The listing builds one solid part. Answer for the finished solid, in the listing's coordinates (mm). A direction names the side the tool comes from. Give positions to 0.01 mm unless a question says otherwise; leave off trailing zeros. Write each loop counter-clockwise with the first axis right and the second up, starting at its lowest first coordinate (ties: lowest second). Pieces come first, ordered by that corner, then holes. Notation, with made-up numbers: M 42,-9.5 L 64,-9.5 A17 ccw 64,1.5 Z; hole C 47,-19 d3. An arc over 180 degrees is marked long. Answer as a JSON object with one key per item and string values.
```python
from build123d import *

# Parameters (mm, degrees)
SKETCH1_W                 = 30
SKETCH1_H                 = 28
SKETCH1_R                 = 11
BOSS_EXTRUDE1_DEPTH       = 7
SKETCH2_W                 = 5
SKETCH2_H                 = 2.5
BOSS_EXTRUDE2_DEPTH       = 13
CHAMFER2_SIZE             = 2
BOSS_EXTRUDE6_DEPTH       = 2.5
CHAMFER3_SIZE             = 2
CHAMFER4_SIZE             = 2
BOSS_EXTRUDE4_DEPTH       = 2.5
CHAMFER6_SIZE             = 2.5
CHAMFER7_SIZE             = 7
CHAMFER7_SIZE_2           = 13.165085257
SKETCH7_R                 = 1.5
CUT_EXTRUDE2_DEPTH        = 6.4
CUT_EXTRUDE3_START        = -3
SKETCH9_R                 = 1.5
CUT_EXTRUDE3_DEPTH        = 3
SKETCH10_W                = 5.5
SKETCH10_H                = 3
CUT_EXTRUDE4_DEPTH        = 5.6
CUT_EXTRUDE5_START        = -30
SKETCH10_2_W              = 5.5
SKETCH10_2_H              = 3
CUT_EXTRUDE5_DEPTH        = 5.6
F_1_0MM_DOWEL_HOLE1_D     = 3
F_1_0MM_DOWEL_HOLE1_DEPTH = 7.098709071
F_1_0MM_DOWEL_HOLE1_TIP   = 0.901290929
BOSS_EXTRUDE7_START       = 3.5
SKETCH17_R                = 1.5
BOSS_EXTRUDE7_DEPTH       = 3.5


with BuildPart() as part:
    # Sketch1 → Boss-Extrude1 (new body)
    with BuildSketch(Plane.XY):
        Rectangle(SKETCH1_W, SKETCH1_H)
        Circle(SKETCH1_R, mode=Mode.SUBTRACT)
    extrude(amount=BOSS_EXTRUDE1_DEPTH)

    # Sketch2 → Boss-Extrude2 (add)
    with BuildSketch(Plane(origin=(0, 0, 0), x_dir=(-1, 0, 0), z_dir=(0, 0, -1))):
        with Locations((-12.5, -12.75)):
            Rectangle(SKETCH2_W, SKETCH2_H)
        with Locations((12.5, -12.75)):
            Rectangle(SKETCH2_W, SKETCH2_H)
    extrude(amount=BOSS_EXTRUDE2_DEPTH)

    # Chamfer2
    chamfer2_edges = [part.edges().sort_by_distance(p)[0] for p in [
        (-10, -12.75, 0),
        (10, -12.75, 0),
    ]]
    chamfer(chamfer2_edges, length=CHAMFER2_SIZE)

    # Sketch5 → Boss-Extrude6 (add)
    with BuildSketch(Plane.XZ.offset(14)):
        Polygon((-10, -2), (-10, -7.5), (10, -7.5), (10, -2), (8, 0), (-8, 0), align=None)
    extrude(amount=-BOSS_EXTRUDE6_DEPTH)

    # Chamfer3
    chamfer3_edges = [part.edges().sort_by_distance(p)[0] for p in [
        (15, 0, 7),
    ]]
    chamfer(chamfer3_edges, length=CHAMFER3_SIZE)

    # Chamfer4
    chamfer4_edges = [part.edges().sort_by_distance(p)[0] for p in [
        (-15, 0, 7),
    ]]
    chamfer(chamfer4_edges, length=CHAMFER4_SIZE)

    # Sketch4 → Boss-Extrude4 (add)
    with BuildSketch(Plane(origin=(0, 0, 0), x_dir=(-1, 0, 0), z_dir=(0, 0, -1))):
        Polygon((-15, 0), (15, 11.5), (15, 14), (-15, 14), align=None)
    extrude(amount=BOSS_EXTRUDE4_DEPTH)

    # Chamfer6
    # the kernel refuses this chamfer: 2.5 mm, written as the material it adds along each edge
    with BuildSketch(Plane(origin=(21.003247512, -2.30124488, 0), x_dir=(-0.3578006820796162, -0.9333930836859554, 0.02749587661058638), z_dir=(-0.9337461173020497, 0.35793601163245237, 0))) as chamfer6_piece_1_section:
        Polygon((CHAMFER6_SIZE * 0.999621916911, -CHAMFER6_SIZE * 0.0274958766106), (-CHAMFER6_SIZE * 0.0274958766106, -CHAMFER6_SIZE * 0.999621916911), (0, 0), align=None)
    chamfer6_piece_1 = extrude(amount=17.263908412, mode=Mode.PRIVATE)
    chamfer6_piece_1 = chamfer6_piece_1 - Plane(origin=(0, 0, -0.835393566), x_dir=(1, 0, 0), z_dir=(0, 0, -1)) * Cylinder(11, 45, mode=Mode.PRIVATE)
    chamfer6_piece_1 = split(chamfer6_piece_1, bisect_by=Plane(origin=(15, -0.113968884, -0.835393566), z_dir=(-1, 0, 0)), keep=Keep.TOP, mode=Mode.PRIVATE)
    add(chamfer6_piece_1)
    with BuildSketch(Plane(origin=(-1.03959441, 6.148511191, 0), x_dir=(-0.35780068207961624, -0.9333930836859554, 0.02749587661058638), z_dir=(-0.9337461173020497, 0.35793601163245237, 0))) as chamfer6_piece_2_section:
        Polygon((CHAMFER6_SIZE * 0.999621916911, -CHAMFER6_SIZE * 0.0274958766106), (-CHAMFER6_SIZE * 0.0274958766106, -CHAMFER6_SIZE * 0.999621916911), (0, 0), align=None)
    chamfer6_piece_2 = extrude(amount=21.380172546, mode=Mode.PRIVATE)
    chamfer6_piece_2 = chamfer6_piece_2 - Plane(origin=(0, 0, -0.851534645), x_dir=(1, 0, 0), z_dir=(0, 0, -1)) * Cylinder(11, 53, mode=Mode.PRIVATE)
    chamfer6_piece_2 = split(chamfer6_piece_2, bisect_by=Plane(origin=(-15, 9.244820467, -0.851534645), z_dir=(1, 0, 0)), keep=Keep.TOP, mode=Mode.PRIVATE)
    add(chamfer6_piece_2)

    # Chamfer7
    # the kernel refuses this chamfer: 13.165085257, 7 mm, written as the material it adds along each edge
    with BuildSketch(Plane(origin=(-15, -11.5, 0), x_dir=(0, 0.9979482451756082, 0.06402577567608186), z_dir=(1, 0, 0))) as chamfer7_piece_1_section:
        Polygon((CHAMFER7_SIZE * 0.997948245176, -CHAMFER7_SIZE * 0.0640257756761), (-CHAMFER7_SIZE_2 * 0.0640257756781, -CHAMFER7_SIZE_2 * 0.997948245208), (0, 0), align=None)
    chamfer7_piece_1 = extrude(amount=30, mode=Mode.PRIVATE)
    chamfer7_piece_1 = chamfer7_piece_1 - Plane(origin=(0, 0, -3.073682767), x_dir=(1, 0, 0), z_dir=(0, 0, -1)) * Cylinder(11, 113, mode=Mode.PRIVATE)
    chamfer7_piece_1 = split(chamfer7_piece_1, bisect_by=Plane(origin=(-10, -8.887755394, -3.073682767), z_dir=(-1, 0, 0)), keep=Keep.TOP, mode=Mode.PRIVATE)
    chamfer7_piece_1 = split(chamfer7_piece_1, bisect_by=Plane(origin=(-12.500128058, -8.887755394, -7.5), z_dir=(0, 0, 1)), keep=Keep.TOP, mode=Mode.PRIVATE)
    add(chamfer7_piece_1)
    with BuildSketch(Plane(origin=(-15, -11.5, 0), x_dir=(0, 0.9979482451756082, 0.06402577567608186), z_dir=(1, 0, 0))) as chamfer7_piece_2_section:
        Polygon((CHAMFER7_SIZE * 0.997948245176, -CHAMFER7_SIZE * 0.0640257756761), (-CHAMFER7_SIZE_2 * 0.0640257756781, -CHAMFER7_SIZE_2 * 0.997948245208), (0, 0), align=None)
    chamfer7_piece_2 = extrude(amount=30, mode=Mode.PRIVATE)
    chamfer7_piece_2 = split(chamfer7_piece_2, bisect_by=Plane(origin=(-10, -10.721530873, -9.597564575), z_dir=(-1, 0, 0)), keep=Keep.TOP, mode=Mode.PRIVATE)
    chamfer7_piece_2 = split(chamfer7_piece_2, bisect_by=Plane(origin=(-12.5, -10.721530873, -7.5), z_dir=(0, 0, -1)), keep=Keep.TOP, mode=Mode.PRIVATE)
    chamfer7_piece_2 = split(chamfer7_piece_2, bisect_by=Plane(origin=(-12.5, -10.721530873, -13), z_dir=(0, 0, 1)), keep=Keep.TOP, mode=Mode.PRIVATE)
    add(chamfer7_piece_2)
    with BuildSketch(Plane(origin=(-15, -11.5, 0), x_dir=(0, 0.9979482451756082, 0.06402577567608186), z_dir=(1, 0, 0))) as chamfer7_piece_3_section:
        Polygon((CHAMFER7_SIZE * 0.997948245176, -CHAMFER7_SIZE * 0.0640257756761), (-CHAMFER7_SIZE_2 * 0.0640257756781, -CHAMFER7_SIZE_2 * 0.997948245208), (0, 0), align=None)
    chamfer7_piece_3 = extrude(amount=30, mode=Mode.PRIVATE)
    chamfer7_piece_3 = chamfer7_piece_3 - Plane(origin=(0, 0, -3.793876077), x_dir=(1, 0, 0), z_dir=(0, 0, -1)) * Cylinder(11, 113, mode=Mode.PRIVATE)
    chamfer7_piece_3 = split(chamfer7_piece_3, bisect_by=Plane(origin=(-10, -6.598719884, -3.793876077), z_dir=(1, 0, 0)), keep=Keep.TOP, mode=Mode.PRIVATE)
    chamfer7_piece_3 = split(chamfer7_piece_3, bisect_by=Plane(origin=(-9.499486782, -6.598719884, -7.5), z_dir=(0, 0, 1)), keep=Keep.TOP, mode=Mode.PRIVATE)
    chamfer7_piece_3 = split(chamfer7_piece_3, bisect_by=Plane(origin=(10, -6.598719884, -3.793876077), z_dir=(-1, 0, 0)), keep=Keep.TOP, mode=Mode.PRIVATE)
    add(chamfer7_piece_3)
    with BuildSketch(Plane(origin=(-15, -11.5, 0), x_dir=(0, 0.9979482451756082, 0.06402577567608186), z_dir=(1, 0, 0))) as chamfer7_piece_4_section:
        Polygon((CHAMFER7_SIZE * 0.997948245176, -CHAMFER7_SIZE * 0.0640257756761), (-CHAMFER7_SIZE_2 * 0.0640257756781, -CHAMFER7_SIZE_2 * 0.997948245208), (0, 0), align=None)
    chamfer7_piece_4 = extrude(amount=30, mode=Mode.PRIVATE)
    chamfer7_piece_4 = split(chamfer7_piece_4, bisect_by=Plane(origin=(12.5, -10.721530873, -7.5), z_dir=(0, 0, -1)), keep=Keep.TOP, mode=Mode.PRIVATE)
    chamfer7_piece_4 = split(chamfer7_piece_4, bisect_by=Plane(origin=(10, -10.721530873, -9.597564575), z_dir=(1, 0, 0)), keep=Keep.TOP, mode=Mode.PRIVATE)
    chamfer7_piece_4 = split(chamfer7_piece_4, bisect_by=Plane(origin=(12.5, -10.721530873, -13), z_dir=(0, 0, 1)), keep=Keep.TOP, mode=Mode.PRIVATE)
    add(chamfer7_piece_4)
    with BuildSketch(Plane(origin=(-15, -11.5, 0), x_dir=(0, 0.9979482451756082, 0.06402577567608186), z_dir=(1, 0, 0))) as chamfer7_piece_5_section:
        Polygon((CHAMFER7_SIZE * 0.997948245176, -CHAMFER7_SIZE * 0.0640257756761), (-CHAMFER7_SIZE_2 * 0.0640257756781, -CHAMFER7_SIZE_2 * 0.997948245208), (0, 0), align=None)
    chamfer7_piece_5 = extrude(amount=30, mode=Mode.PRIVATE)
    chamfer7_piece_5 = chamfer7_piece_5 - Plane(origin=(0, 0, -3.073682766), x_dir=(1, 0, 0), z_dir=(0, 0, -1)) * Cylinder(11, 113, mode=Mode.PRIVATE)
    chamfer7_piece_5 = split(chamfer7_piece_5, bisect_by=Plane(origin=(12.500128057, -8.887755394, -7.5), z_dir=(0, 0, 1)), keep=Keep.TOP, mode=Mode.PRIVATE)
    chamfer7_piece_5 = split(chamfer7_piece_5, bisect_by=Plane(origin=(10, -8.887755394, -3.073682766), z_dir=(1, 0, 0)), keep=Keep.TOP, mode=Mode.PRIVATE)
    add(chamfer7_piece_5)

    # Sketch7 → Cut-Extrude2 (cut)
    with BuildSketch(Plane.XZ.offset(14)):
        with Locations(Location((-11, 2.5, 0), (0, 0, 270))):
            Circle(SKETCH7_R)
        with Locations(Location((11, 2.5, 0), (0, 0, 270))):
            Circle(SKETCH7_R)
    extrude(amount=-CUT_EXTRUDE2_DEPTH, mode=Mode.SUBTRACT)

    # Sketch9 → Cut-Extrude3 (cut)
    # profile 1 of 2: a face of its own
    with BuildSketch(Plane.XZ.offset(14).offset(CUT_EXTRUDE3_START)):
        Polygon((7.824573519, 2.5), (9.41228676, -0.25), (12.58771324, -0.25), (14.175426481, 2.5), (12.58771324, 5.25), (9.41228676, 5.25), align=None)
        with Locations(Location((11, 2.5, 0), (0, 0, 270))):
            Circle(SKETCH9_R, mode=Mode.SUBTRACT)
    # profile 2 of 2: a face of its own
    with BuildSketch(Plane.XZ.offset(14).offset(CUT_EXTRUDE3_START)):
        Polygon((-7.824573519, 2.5), (-9.41228676, 5.25), (-12.58771324, 5.25), (-14.175426481, 2.5), (-12.58771324, -0.25), (-9.41228676, -0.25), align=None)
        with Locations(Location((-11, 2.5, 0), (0, 0, 270))):
            Circle(SKETCH9_R, mode=Mode.SUBTRACT)
    extrude(amount=-CUT_EXTRUDE3_DEPTH, mode=Mode.SUBTRACT)

    # Sketch10 → Cut-Extrude4 (cut)
    with BuildSketch(Plane(origin=(15, 0, 0), x_dir=(0, 0, -1), z_dir=(1, 0, 0))):
        with Locations((-2.5, -9.5)):
            Rectangle(SKETCH10_W, SKETCH10_H)
    extrude(amount=-CUT_EXTRUDE4_DEPTH, mode=Mode.SUBTRACT)

    # Sketch10<2> → Cut-Extrude5 (cut)
    with BuildSketch(Plane(origin=(15, 0, 0), x_dir=(0, 0, -1), z_dir=(1, 0, 0)).offset(CUT_EXTRUDE5_START)):
        with Locations((-2.5, -9.5)):
            Rectangle(SKETCH10_2_W, SKETCH10_2_H)
    extrude(amount=CUT_EXTRUDE5_DEPTH, mode=Mode.SUBTRACT)

    # Ø1.0mm Dowel Hole1
    with Locations(Plane(origin=(0, 14, 0), x_dir=(1, 0, 0), z_dir=(0, 1, 0))):
        with Locations((-11.6, -1.25), (11.6, -1.25)):
            Hole(F_1_0MM_DOWEL_HOLE1_D / 2, depth=F_1_0MM_DOWEL_HOLE1_DEPTH)
            with Locations((0, 0, -(F_1_0MM_DOWEL_HOLE1_DEPTH + F_1_0MM_DOWEL_HOLE1_TIP / 2))):  # 118° drill point
                Cone(0, F_1_0MM_DOWEL_HOLE1_D / 2, F_1_0MM_DOWEL_HOLE1_TIP, mode=Mode.SUBTRACT)

    # Sketch17 → Boss-Extrude7 (add)
    with BuildSketch(Plane.XZ.offset(14).offset(BOSS_EXTRUDE7_START)):
        Polygon((13, 7), (-13, 7), (-15, 5), (-15, -13), (-10, -13), (-10, -7.5), (10, -7.5), (10, -13), (15, -13), (15, 5), align=None)
        with Locations(Location((-11, 2.5, 0), (0, 0, 270))):
            Circle(SKETCH17_R, mode=Mode.SUBTRACT)
        with Locations(Location((11, 2.5, 0), (0, 0, 270))):
            Circle(SKETCH17_R, mode=Mode.SUBTRACT)
    extrude(amount=-BOSS_EXTRUDE7_DEPTH)


solid = part.part
```
1. For faces 5 (the flat face through (12.97, -0.58, -1.23)), 6 (the flat face through (0, -13, -7.5)), 7 (the flat face through (11.83, -7.91, -6.41)), 8 (the flat face through (4, 9, -2.5)), determine the directions among +Z, -Z, +X, -X, +Y, -Y from which every point of the face is accessible in a straight line to the end or side of a thin tool.
Verdict:
{"face 5": "-Z, -X", "face 6": "-Z, +Y, -Y", "face 7": "-Z, +X, -X", "face 8": "-Z, +X, -X, +Y"}
2. A cutting plane is placed at A-A, the plane x = 0. Give the vertices of the cut face in (y, z), plus the area to 3 significant figures.
Verdict:
{"outline": "M -17.5,-7.5 L -11,-7.5 L -11,7 L -17.5,7 Z; M 5.75,-2.5 L 14,-2.5 L 14,7 L 11,7 L 11,0 L 5.75,0 Z", "area": "136 mm2"}
3. Flat-ended cylindrical pins translate along their axes: pin 1 (1.6 mm diameter, centred on x = -11, z = 3, fed in from -Y); pin 2 (1.8 mm diameter, centred on x = 11.6, z = 1.25, fed in from +Y); pin 3 (2.5 mm diameter, centred on x = -11.5, y = -9, fed in from -Z). Find the tip coordinate at first contact, or state that the pin passes through.
Verdict:
{"pin 1": "stops at y = -7.6", "pin 2": "stops at y = 6.54", "pin 3": "stops at z = -10.81"}
4. A cutting plane is placed at D-D, the plane x = 5.75. Give the vertices of the cut face in (y, z).
Verdict:
{"outline": "M -17.5,-7.5 L -9.38,-7.5 L -9.38,7 L -17.5,7 Z; M 3.55,-2.5 L 14,-2.5 L 14,7 L 9.38,7 L 9.38,0 L 3.55,0 Z"}
5. The mould has two halves that part along Z. Classify faces 1 (the cylindrical face through (-12.33, -7.8, 1.81)), 2 (the flat face through (-14, -2, 6)), 3 (the flat face through (12, -3, 0)), 4 (the flat face through (-12, -10, 5.25)): released by +Z, released by -Z, zero draft, split by the parting line, or undercut.
Verdict:
{"face 1": "undercut", "face 2": "released by +Z", "face 3": "released by -Z", "face 4": "undercut"}
6. Consider line 1 along X through (y, z) = (0, 4.25); line 2 along Z through (x, y) = (11.6, 10.5); line 3 along X through (y, z) = (-15, -12). Determine where each line is inside the solid, lowest interval first.
Verdict:
{"line 1": "x = -15 to -11, 11 to 15", "line 2": "z = -2.5 to -0.25, 2.75 to 7", "line 3": "x = -15 to -10, 10 to 15"}
7. A cutting plane is placed at B-B, the plane z = -8. Give the vertices of the cut face in (x, y).
Verdict:
{"outline": "M -15,-17.5 L -10,-17.5 L -10,-8.75 L -15,-8.75 Z; M 10,-17.5 L 15,-17.5 L 15,-8.75 L 10,-8.75 Z"}
